```python
from build123d import *

# Parameters (mm, degrees)
F1_DEPTH      = 83.82
F2_DEPTH      = 101.6
F2_DEPTH_BACK = 17.78
F4_DEPTH      = 176.022


with BuildPart() as f1:
    # F0 (on Front) → F1 (new body)
    with BuildSketch(Plane.XZ):
        with BuildLine():
            Line((-86.2852931023, -45.4958863556), (86.2852931023, -45.4958863556))
            Line((86.2852931023, -45.4958863556), (86.2852931023, 45.4958863556))
            Line((86.2852931023, 45.4958863556), (45.2049326768, 45.4958863556))
            ThreePointArc((45.2049326768, 45.4958863556), (0, 0.2909536789), (-45.2049326768, 45.4958863556))
            Line((-45.2049326768, 45.4958863556), (-86.2852931023, 45.4958863556))
            Line((-86.2852931023, 45.4958863556), (-86.2852931023, -45.4958863556))
        make_face()
    extrude(amount=-F1_DEPTH)

    # F0 (on Front) → F2 (join, two sides)
    with BuildSketch(Plane.XZ) as f2_sk:
        with BuildLine():
            ThreePointArc((-45.2049326768, 45.4958863556), (0, 0.2909536789), (45.2049326768, 45.4958863556))
            Line((45.2049326768, 45.4958863556), (23.7693889097, 45.4958863556))
            ThreePointArc((23.7693889097, 45.4958863556), (0, 21.726497446), (-23.7693889097, 45.4958863556))
            Line((-23.7693889097, 45.4958863556), (-45.2049326768, 45.4958863556))
        make_face()
    extrude(amount=-F2_DEPTH)
    extrude(f2_sk.sketch, amount=F2_DEPTH_BACK)

    # F3 (on face) → F4 (cut, symmetric)
    with BuildSketch(Plane.XY.offset(45.4958863556)):
        with BuildLine():
            ThreePointArc((-38.6172999535, 41.91), (-55.5423423648, 58.8350424113), (-72.4673847761, 41.91))
            Line((-72.4673847761, 41.91), (-38.6172999535, 41.91))
        make_face()
        with BuildLine():
            ThreePointArc((72.4673847761, 41.91), (55.5423423648, 58.8350424113), (38.6172999535, 41.91))
            Line((38.6172999535, 41.91), (72.4673847761, 41.91))
        make_face()
        with BuildLine():
            Line((72.4673847761, 41.91), (38.6172999535, 41.91))
            ThreePointArc((38.6172999535, 41.91), (55.5423423648, 24.9849575887), (72.4673847761, 41.91))
        make_face()
        with BuildLine():
            Line((-38.6172999535, 41.91), (-72.4673847761, 41.91))
            ThreePointArc((-72.4673847761, 41.91), (-55.5423423648, 24.9849575887), (-38.6172999535, 41.91))
        make_face()
    extrude(amount=F4_DEPTH, both=True, mode=Mode.SUBTRACT)


solid = f1.part
```
Work out the finished part from the listing and answer in its coordinate system (mm). A direction names the side the tool comes from. Give positions to 0.01 mm unless a question says otherwise; leave off trailing zeros. Order: outer loops, then holes, each group sorted by start corner. A loop starts at its lowest first (then second) coordinate and runs counter-clockwise, first axis right, second up. Notation, with made-up numbers: (3.25, 52) - (24.25, 52) arc R26 cw to (24.25, 89) - close; hole circle Ø11 at (48.5, -4.75). An arc over 180 degrees is marked (long way). One line per item, written item: value. Start each with the question number.
1. Section D-D, the plane x = 0 is taken. Write down the section's boundary in (y, z).
2. Section B-B, the plane z = -4 is taken. Write down the section's boundary in (x, y), then the cut area to 3 significant figures.
3. Section A-A, the plane y = 41.91 is taken. Write down the section's boundary in (x, z).
4. Section C-C, the plane z = 36.5 is taken. Write down the section's boundary in (x, y).
5. For a pull along X with two mould halves and no side action, classify faces 4 (the face through (-0.99, -8.77, 0.3)), 5 (the face through (-41, 29, 45.496)), 6 (the face through (-43.07, 30.47, 0.64)) as released by +X, released by -X, zero draft, split by the parting line, or undercut.
6. Consider line 1 (X direction, y = 41.91, z = 1.5); line 2 (X direction, y = 41, z = -19); line 3 (X direction, y = 51, z = 35.5). Determine where each line is inside the solid, lowest interval first.
7. Which of the six approach directions +Z, -Z, +X, -X, +Y, -Y give full straight-line access (tool end or side, diameter ignored) to faces 1 (the face through (86.285, 41, -1)), 2 (the face through (-0.99, 92.59, 0.3)), 3 (the face through (-1, 0, -9))?
8. This flat-tipped pin is pushed along its axis until it touches: pin 1 Ø8 at (x, z) = (66, 16) entering from +Y. Where does it stop, or does it pass through?
Filled sheet:
1. outline: (-17.78, 0.29) - (0, 0.29) - (0, -45.5) - (83.82, -45.5) - (83.82, 0.29) - (101.6, 0.29) - (101.6, 21.73) - (-17.78, 21.73) - close
2. outline: (-86.29, 0) - (86.29, 0) - (86.29, 83.82) - (-86.29, 83.82) - close; hole circle Ø33.85 at (-55.54, 41.91); hole circle Ø33.85 at (55.54, 41.91)
2. area: 12,700 mm²
3. outline: (-86.29, -45.5) - (-72.47, -45.5) - (-72.47, 45.5) - (-86.29, 45.5) - close; (-38.62, -45.5) - (38.62, -45.5) - (38.62, 45.5) - (23.77, 45.5) arc R23.77 cw to (-23.77, 45.5) - (-38.62, 45.5) - close; (72.47, -45.5) - (86.29, -45.5) - (86.29, 45.5) - (72.47, 45.5) - close
4. outline: (-86.29, 0) - (-44.3, 0) - (-44.3, -17.78) - (-22, -17.78) - (-22, 101.6) - (-44.3, 101.6) - (-44.3, 83.82) - (-86.29, 83.82) - close; (22, -17.78) - (44.3, -17.78) - (44.3, 0) - (86.29, 0) - (86.29, 83.82) - (44.3, 83.82) - (44.3, 101.6) - (22, 101.6) - close; hole circle Ø33.85 at (-55.54, 41.91); hole circle Ø33.85 at (55.54, 41.91)
5. face 4: split by the parting line
5. face 5: zero draft
5. face 6: undercut
6. line 1: -86.29 to -72.47, -38.62 to 38.62, 72.47 to 86.29
6. line 2: -86.29 to -72.44, -38.64 to 38.64, 72.44 to 86.29
6. line 3: -86.29 to -69.82, -41.27 to -21.57, 21.57 to 41.27, 69.82 to 86.29
7. face 1: +Z, -Z, +X, +Y, -Y
7. face 2: -Z, +Y
7. face 3: -Z, -Y
8. pin 1: y = 83.82
